Read the model definition and answer for the solid it produces. Units are mm, in the model's axes. A direction names the side the tool comes from. Coordinates: 2 decimals unless noted, no trailing zeros. Write each loop counter-clockwise with the first axis right and the second up, starting at its lowest first coordinate (ties: lowest second). Pieces come first, ordered by that corner, then holes. Notation, with made-up numbers: (-13.75, -20.75) -> (30.25, -20.75) arc R33 cw to (30.25, 18.25) -> close; hole circle Ø3 at (58, 1.5). An arc over 180 degrees is marked (long way). Answer as a JSON object with one key per item and string values. Group by question number.
(1) Straight lines are drawn through the part: L1, parallel to Y at x = 55, z = 43; L2, parallel to Z at x = -5, y = 25. For each, find the intervals that lie inside material, in ascending order.
(2) Which of the six approach directions +Z, -Z, +X, -X, +Y, -Y give full straight-line access (tool end or side, diameter ignored) to faces 4 (the face through (55, -50, 28)), 5 (the face through (21.886, -14.51, 10.437)), 6 (the face through (-50, 55, 28))?
(3) For a pull along X with two mould halves and no side action, classify faces 1 (the face through (-8.8, 43.3, 10.4)), 2 (the face through (50, 55, 28)), 3 (the face through (-1, -1, 0)) as +X half, -X half, draft (parallel to the pull), parting line (faces both ways), or undercut.
(4) Find section B-B (y = -32.5). Give the vertices of the cut face in (x, z).
(5) Flat-ended cylindrical pins translate along their axes: P1, Ø3, axis at x = -23.5, y = -9.5, coming from the +Z side; P2, Ø2, axis at x = -44.5, y = -17.5, coming from the +Z side; P3, Ø2, axis at x = 55, y = 55, coming from the +Z side; P4, Ø5, axis at x = -11, y = -36.5, coming from the -Z side. Find the tip coordinate at first contact, or state that the pin passes through.
(6) Find section A-A (z = 18). Give the vertices of the cut face in (x, y), then the cut area to 3 significant figures.
from build123d import *

# Parameters (mm, degrees)
SKETCH1_W                                  = 120
SKETCH1_H                                  = 120
BOSS_EXTRUDE1_DEPTH                        = 6
SKETCH2_W                                  = 10
SKETCH2_H                                  = 10
BOSS_EXTRUDE2_DEPTH                        = 45
SKETCH4_R                                  = 1.25
CUT_EXTRUDE1_DEPTH                         = 14
MIRROR1_AT_THE_SECOND_PLANE_COPY_1_SKETC_R = 1.25
MIRROR1_AT_THE_SECOND_PLANE_COPY_1_DEPTH   = 14
SKETCH5_R                                  = 3.15
BOSS_EXTRUDE4_DEPTH                        = 9
SKETCH7_R                                  = 1.15
CUT_EXTRUDE2_DEPTH                         = 9


with BuildPart() as part:
    # Sketch1 → Boss-Extrude1 (new body)
    with BuildSketch(Plane(origin=(0, 0, 0), x_dir=(0, 1, 0), z_dir=(0, 0, 1))):
        Rectangle(SKETCH1_W, SKETCH1_H)
    extrude(amount=BOSS_EXTRUDE1_DEPTH)

    # Sketch2 → Boss-Extrude2 (add)
    with BuildSketch(Plane.XY.offset(6)):
        with Locations((-55, 55)):
            Rectangle(SKETCH2_W, SKETCH2_H)
        with Locations((55, 55)):
            Rectangle(SKETCH2_W, SKETCH2_H)
        with Locations((55, -55)):
            Rectangle(SKETCH2_W, SKETCH2_H)
        with Locations((-55, -55)):
            Rectangle(SKETCH2_W, SKETCH2_H)
    extrude(amount=BOSS_EXTRUDE2_DEPTH)

    # Sketch4 → Cut-Extrude1 (cut)
    with BuildSketch(Plane.XY.offset(51)):
        with Locations((-55, 55)):
            Circle(SKETCH4_R)
    cut_extrude1 = extrude(amount=-CUT_EXTRUDE1_DEPTH, mode=Mode.SUBTRACT)

    # Mirror1: Cut-Extrude1 across plane
    add(cut_extrude1.mirror(Plane.ZX), mode=Mode.SUBTRACT)

    # Mirror1 at the second plane: Cut-Extrude1 across plane
    add(cut_extrude1.mirror(Plane(origin=(0, 0, 0), x_dir=(0, 0, 1), z_dir=(1, 0, 0))), mode=Mode.SUBTRACT)

    # Mirror1 at the second plane copy 1 sketc → Mirror1 at the second plane copy 1 (cut)
    with BuildSketch(Plane(origin=(0, 0, 51), x_dir=(-1, 0, 0), z_dir=(0, 0, 1))):
        with Locations((-55, 55)):
            Circle(MIRROR1_AT_THE_SECOND_PLANE_COPY_1_SKETC_R)
    extrude(amount=-MIRROR1_AT_THE_SECOND_PLANE_COPY_1_DEPTH, mode=Mode.SUBTRACT)

    # Sketch5 → Boss-Extrude4 (add)
    with BuildSketch(Plane.XY.offset(6)):
        with Locations(Location((-9.440556716, 40.216124503, 0), (0, 0, 180))):
            Circle(SKETCH5_R)
        with Locations(Location((-24.680556716, -10.583875497, 0), (0, 0, 180))):
            Circle(SKETCH5_R)
        with Locations(Location((23.579443284, -11.853875497, 0), (0, 0, 180))):
            Circle(SKETCH5_R)
    extrude(amount=BOSS_EXTRUDE4_DEPTH)

    # Sketch7 → Cut-Extrude2 (cut)
    with BuildSketch(Plane(origin=(0, 0, 15), x_dir=(0, -1, 0), z_dir=(0, 0, 1))):
        with Locations(Location((-40.216124503, -9.440556716, 0), (0, 0, 90))):
            Circle(SKETCH7_R)
        with Locations(Location((11.853875497, 23.579443284, 0), (0, 0, 90))):
            Circle(SKETCH7_R)
        with Locations(Location((10.583875497, -24.680556716, 0), (0, 0, 90))):
            Circle(SKETCH7_R)
    extrude(amount=-CUT_EXTRUDE2_DEPTH, mode=Mode.SUBTRACT)


solid = part.part
Results below:
{
 "1": {"L1": "y = -60 to -56.25, -53.75 to -50, 50 to 53.75, 56.25 to 60", "L2": "z = 0 to 6"},
 "2": {"face 4": "+Z, +X, -X", "face 5": "+Z", "face 6": "+Z, +Y, -Y"},
 "3": {"face 1": "parting line", "face 2": "undercut", "face 3": "draft"},
 "4": {"outline": "(-60, 0) -> (60, 0) -> (60, 6) -> (-60, 6) -> close"},
 "5": {"P1": "stops at z = 15", "P2": "stops at z = 6", "P3": "stops at z = 37", "P4": "stops at z = 0"},
 "6": {"outline": "(-60, -60) -> (-50, -60) -> (-50, -50) -> (-60, -50) -> close; (-60, 50) -> (-50, 50) -> (-50, 60) -> (-60, 60) -> close; (50, -60) -> (60, -60) -> (60, -50) -> (50, -50) -> close; (50, 50) -> (60, 50) -> (60, 60) -> (50, 60) -> close", "area": "400 mm2"}
}
